from build123d import *

# Parameters (mm, degrees)
F0_R     = 30.32125
F1_DEPTH = 6.35
F2_R     = 0.381


with BuildPart() as f1:
    # F0 (on Front) → F1 (new body)
    with BuildSketch(Plane.XZ):
        Circle(F0_R)
        with BuildLine():
            ThreePointArc((-2.921, -22.928688), (-16.344066, -16.344066), (-22.928688, -2.921))
            Line((-22.928688, -2.921), (-20.6375, -2.921))
            Line((-20.6375, -2.921), (-20.6375, 2.921))
            Line((-20.6375, 2.921), (-22.928688, 2.921))
            ThreePointArc((-22.928688, 2.921), (-16.344066, 16.344066), (-2.921, 22.928688))
            Line((-2.921, 22.928688), (-2.921, 20.6375))
            Line((-2.921, 20.6375), (2.921, 20.6375))
            Line((2.921, 20.6375), (2.921, 22.928688))
            ThreePointArc((2.921, 22.928688), (16.344066, 16.344066), (22.928688, 2.921))
            Line((22.928688, 2.921), (20.6375, 2.921))
            Line((20.6375, 2.921), (20.6375, -2.921))
            Line((20.6375, -2.921), (22.928688, -2.921))
            ThreePointArc((22.928688, -2.921), (16.344066, -16.344066), (2.921, -22.928688))
            Line((2.921, -22.928688), (2.921, -20.6375))
            Line((2.921, -20.6375), (-2.921, -20.6375))
            Line((-2.921, -20.6375), (-2.921, -22.928688))
        make_face(mode=Mode.SUBTRACT)
    extrude(amount=F1_DEPTH)

    # F2
    f2_edges = [f1.edges().sort_by_distance(p)[0] for p in [
        (-2.921, -3.175, 20.6375),
        (-2.921, -3.175, 22.928688),
        (2.921, -3.175, 20.6375),
        (-20.6375, -3.175, -2.921),
        (22.928688, -3.175, -2.921),
        (20.6375, -3.175, -2.921),
        (20.6375, -3.175, 2.921),
        (-2.921, -3.175, -20.6375),
        (2.921, -3.175, -20.6375),
        (-2.921, -3.175, -22.928688),
        (-20.6375, -3.175, 2.921),
        (22.928688, -3.175, 2.921),
        (2.921, -3.175, 22.928688),
        (-22.928688, -3.175, -2.921),
        (2.921, -3.175, -22.928688),
        (-22.928688, -3.175, 2.921),
    ]]
    fillet(f2_edges, radius=F2_R)


solid = f1.part
Geometry check sheet. Reference: the model listing, model coordinates, mm. A direction names the side the tool comes from. Coordinates: 2 decimals unless noted, no trailing zeros. Order: outer loops, then holes, each group sorted by start corner. A loop starts at its lowest first (then second) coordinate and runs counter-clockwise, first axis right, second up. Notation, with made-up numbers: (-16, -20) - (12, -20) arc R18 ccw to (12, -9) - close; hole circle Ø8 at (0.5, -17). An arc over 180 degrees is marked (long way). Answer in a Markdown table with one row per item. Add a question column.
1) Cross-section at B-B, the plane x = 0. Record the cut outline in (y, z), then the cut area to 3 significant figures.
2) Cross-section at D-D, the plane z = 25.5. Record the cut outline in (x, y).
3) Cross-section at C-C, the plane z = 19. Record the cut outline in (x, y).
4) Set-up check for faces 4 (the flat face through (-21, 0, 0)), 5 (the flat face through (-2.921, -3, -22)): record each of +Z, -Z, +X, -X, +Y, -Y from which the full face is reachable in a straight line by a thin tool's end or side.
5) Material ranges on line 1 along X through (y, z) = (-5.5, -21); line 2 along Z through (x, y) = (-10, -5.75); line 3 along Z through (x, y) = (4.5, -0.5), recorded low to high. Write a range as [from, to].
6) Gauge pin test, flat ends, axial feed: P1, Ø3, axis at y = -3.5, z = -5.5, coming from the +X side; P2, Ø1.6, axis at x = 21.5, y = -3, coming from the +Z side; P3, Ø1.2, axis at x = -21.5, y = -3, coming from the +Z side. Record the tip position at first contact, or that the pin passes through.
7) Release check for a two-part mould opening along X. For faces 1 (the flat face through (-22, -3, -2.921)), 2 (the cylindrical face through (28.92, -3.13, 9.11)), 3 (the flat face through (-21, -6.35, 0)) record: +X half, -X half, draft (parallel to the pull), parting line (faces both ways), or undercut.
Check result:
| question | item | result |
|---|---|---|
| 1 | outline | (-6.35, -30.32) - (0, -30.32) - (0, -20.64) - (-6.35, -20.64) - close; (-6.35, 20.64) - (0, 20.64) - (0, 30.32) - (-6.35, 30.32) - close |
| 1 | area | 123 mm² |
| 2 | outline | (-16.41, -6.35) - (16.41, -6.35) - (16.41, 0) - (-16.41, 0) - close |
| 3 | outline | (-23.63, -6.35) - (-13.16, -6.35) - (-13.16, 0) - (-23.63, 0) - close; (13.16, -6.35) - (23.63, -6.35) - (23.63, 0) - (13.16, 0) - close |
| 4 | face 4 | +Z, -Z, +X, -X, +Y |
| 4 | face 5 | +Y, -Y |
| 5 | line 1 | x = [-21.87, -9.66], [-2.92, 2.92], [9.66, 21.87] |
| 5 | line 2 | z = [-28.62, -20.84], [20.84, 28.62] |
| 5 | line 3 | z = [-29.99, -22.67], [22.67, 29.99] |
| 6 | P1 | stops at x = 30.06 |
| 6 | P2 | stops at z = 22.16 |
| 6 | P3 | stops at z = 21.97 |
| 7 | face 1 | undercut |
| 7 | face 2 | parting line |
| 7 | face 3 | draft |
